CAD build for the part. Positions are in the model's coordinates, mm. A direction names the side the tool comes from. Round coordinates to 2 decimals unless told otherwise and drop trailing zeros. Order: outer loops, then holes, each group sorted by start corner. A loop starts at its lowest first (then second) coordinate and runs counter-clockwise, first axis right, second up. Notation, with made-up numbers: M -8.5,31 L 19.5,31 A23 ccw 19.5,41 Z; hole C -10,3 d2. An arc over 180 degrees is marked long. Answer as a JSON object with one key per item and string values. Group by question number.
```python
from build123d import *

# Parameters (mm, degrees)
SKETCH1_W           = 6.35
SKETCH1_H           = 25.4
BOSS_EXTRUDE1_DEPTH = 3.0226
SKETCH4_W           = 2.667
SKETCH4_H           = 6.096
CUT_EXTRUDE2_DEPTH  = 6.0452
SKETCH5_W           = 2.54
SKETCH5_H           = 27.94
BOSS_EXTRUDE2_DEPTH = 6.0452


with BuildPart() as part:
    # Sketch1 → Boss-Extrude1 (new, symmetric)
    with BuildSketch(Plane(origin=(0, 0, 0), x_dir=(1, 0, 0), z_dir=(0, 1, 0))):
        Polygon((0, -39.116), (0, 39.116), (-44.577, 39.116), (-44.577, 12.7), (-44.577, -12.7), (-44.577, -39.116), align=None)
        with Locations((-47.752, 0)):
            Rectangle(SKETCH1_W, SKETCH1_H)
        Polygon((44.577, 39.116), (0, 39.116), (0, -39.116), (44.577, -39.116), (44.577, -12.7), (44.577, 12.7), align=None)
        with Locations((47.752, 0)):
            Rectangle(SKETCH1_W, SKETCH1_H)
    extrude(amount=BOSS_EXTRUDE1_DEPTH, both=True)

    # Sketch4 → Cut-Extrude2 (cut)
    with BuildSketch(Plane(origin=(0, 3.0226, 0), x_dir=(1, 0, 0), z_dir=(0, 1, 0))):
        with Locations((-40.1955, -31.75)):
            Rectangle(SKETCH4_W, SKETCH4_H)
        with Locations((-40.1955, -19.05)):
            Rectangle(SKETCH4_W, SKETCH4_H)
        with Locations((-40.1955, -6.35)):
            Rectangle(SKETCH4_W, SKETCH4_H)
        with Locations((-40.1955, 6.35)):
            Rectangle(SKETCH4_W, SKETCH4_H)
        with Locations((-40.1955, 19.05)):
            Rectangle(SKETCH4_W, SKETCH4_H)
        with Locations((-40.1955, 31.75)):
            Rectangle(SKETCH4_W, SKETCH4_H)
        with Locations((40.1955, -19.05)):
            Rectangle(SKETCH4_W, SKETCH4_H)
        with Locations((40.1955, -6.35)):
            Rectangle(SKETCH4_W, SKETCH4_H)
        with Locations((40.1955, 6.35)):
            Rectangle(SKETCH4_W, SKETCH4_H)
        with Locations((40.1955, 19.05)):
            Rectangle(SKETCH4_W, SKETCH4_H)
        with Locations((40.1955, 31.75)):
            Rectangle(SKETCH4_W, SKETCH4_H)
        with Locations((40.1955, -31.75)):
            Rectangle(SKETCH4_W, SKETCH4_H)
    extrude(amount=-CUT_EXTRUDE2_DEPTH, mode=Mode.SUBTRACT)

    # Sketch5 → Boss-Extrude2 (add)
    with BuildSketch(Plane(origin=(0, 3.0226, 0), x_dir=(1, 0, 0), z_dir=(0, 1, 0))):
        with Locations((-52.197, 0)):
            Rectangle(SKETCH5_W, SKETCH5_H)
        with Locations((52.197, 0)):
            Rectangle(SKETCH5_W, SKETCH5_H)
    extrude(amount=-BOSS_EXTRUDE2_DEPTH)


solid = part.part
```
Item 1: Flat gauge pin, fed straight in: pin 1 Ø3 at (y, z) = (-1, -31) entering from -X. Where does the tip first touch, or does it go through?
Item 2: Cut at B-B, the plane z = -30. Give the cut face in (x, y), and give its area (3 significant figures).
Item 3: 3-axis set-ups, long thin cutter, end or side, ignore diameter. For faces 4 (the face through (53.467, 0, 0)), 5 (the face through (-41.529, 0, -6)), 6 (the face through (52, 0, 13.97)), 7 (the face through (52, 0, -13.97)): which of +Z, -Z, +X, -X, +Y, -Y reach the whole face in a straight line?
Item 4: Drill centre lines: line 1 (X direction, y = 1.75, z = 9); line 2 (X direction, y = -1.5, z = -19.5); line 3 (Z direction, x = 47, y = 0). Where is each one in solid material? Low to high. Write a range as [from, to].
Item 5: Two-plate mould, pull along Z, no slides. Class faces 1 (the face through (-40, 0, 28.702)), 2 (the face through (-53.467, 0, 0)), 3 (the face through (-48, 0, -12.7)): +Z half, -Z half, draft (parallel to the pull), parting line (faces both ways), or undercut.
Item 6: Cut at C-C, the plane y = -0.75. Give the number of separate pieces and of enclosed holes in the cut face, and give its area (3 significant figures).
Item 7: Cut at A-A, the plane z = 5. Give the cut face in (x, y).
Response values:
{
 "1": {"pin 1": "x = -44.58"},
 "2": {"outline": "M -44.58,-3.02 L -41.53,-3.02 L -41.53,3.02 L -44.58,3.02 Z; M -38.86,-3.02 L 38.86,-3.02 L 38.86,3.02 L -38.86,3.02 Z; M 41.53,-3.02 L 44.58,-3.02 L 44.58,3.02 L 41.53,3.02 Z", "area": "507 mm^2"},
 "3": {"face 4": "+Z, -Z, +X, +Y, -Y", "face 5": "+Y, -Y", "face 6": "+Z, +X, +Y, -Y", "face 7": "-Z, +X, +Y, -Y"},
 "4": {"line 1": "[-53.47, -41.53], [-38.86, 38.86], [41.53, 53.47]", "line 2": "[-44.58, -41.53], [-38.86, 38.86], [41.53, 44.58]", "line 3": "[-12.7, 12.7]"},
 "5": {"face 1": "undercut", "face 2": "draft", "face 3": "-Z half"},
 "6": {"separate pieces": "1", "enclosed holes": "12", "area": "7,240 mm^2"},
 "7": {"outline": "M -53.47,-3.02 L -41.53,-3.02 L -41.53,3.02 L -53.47,3.02 Z; M -38.86,-3.02 L 38.86,-3.02 L 38.86,3.02 L -38.86,3.02 Z; M 41.53,-3.02 L 53.47,-3.02 L 53.47,3.02 L 41.53,3.02 Z"}
}
